Read the model definition and answer for the solid it produces. Units are mm, in the model's axes. Coordinates: 2 decimals unless noted, no trailing zeros. Order: outer loops, then holes, each group sorted by start corner. A loop starts at its lowest first (then second) coordinate and runs counter-clockwise, first axis right, second up. Notation, with made-up numbers: M 62,66.25 L 85,66.25 A22 ccw 85,74.25 Z; hole C 23.25,-9 d4. An arc over 180 degrees is marked long. One line per question, with ' | ' between items. Start each with the question number.
1) Given P1, Ø6, axis at x = -5.5, z = 50.5, coming from the +Y side; P2, Ø5, axis at x = 7.5, z = 30, coming from the -Y side; P3, Ø6, axis at x = 7.5, z = 32, coming from the +Y side, each flat-ended and moving along its own axis, determine where each tip first touches the part or whether it passes through.
2) Find section A-A, the plane x = 0. Write down the section's boundary in (y, z), plus the area to 3 significant figures.
3) Find section C-C, the plane z = 16. Write down the section's boundary in (x, y).
4) The mould has two halves that part along X. Classify faces 1 (the face through (2.994, -22.804, 30.42)), 2 (the face through (23.846, -7.509, 29.58)), 3 (the face through (22.1, -7.3, 60)): +X half, -X half, draft (parallel to the pull), parting line (faces both ways), or undercut.
5) Consider probe 1 along Y at (x, z) = (0, 38.5); probe 2 along Y at (x, z) = (14, 57.5); probe 3 along X at (y, z) = (13.5, 19.5). Determine where each line is inside the solid, lowest interval first.
Autodesk Fusion 360 part; units mm, degrees
sketch "スケッチ1" plane through (0, 0, 0) normal (0, 0, 1) x (1, 0, 0)
  circle A0 centre (0, 0) radius 25
  circle A1 centre (0, 0) radius 22.5
  dimension "d1" = 45
extrude "押し出し1" add sketch "スケッチ1" along normal blind 70
sketch "スケッチ2" plane through (0, 0, 70) normal (0, 0, 1) x (-1, 0, 0)
  circle A0 centre (0, 0) radius 22.5
  circle A1 centre (0, 0) radius 25
  circle A2 centre (0, 0) radius 23
extrude "押し出し2" cut sketch "スケッチ2" against normal blind 75 contours A2
extrude "押し出し3" cut 1 faces at (24.1546, -2.3847, 70) along direction (0, 0, -1) blind 10
Report:
1) P1: stops at y = 24.87 | P2: stops at y = -24.49 | P3: stops at y = 24.59
2) outline: M -25,0 L -23,0 L -23,60 L -25,60 Z; M 23,0 L 25,0 L 25,60 L 23,60 Z | area: 240 mm^2
3) outline: C 0,0 d50; hole C 0,0 d46
4) face 1: undercut | face 2: parting line | face 3: draft
5) probe 1: y = -25 to -23, 23 to 25 | probe 2: y = -20.71 to -18.25, 18.25 to 20.71 | probe 3: x = -21.04 to -18.62, 18.62 to 21.04
